from build123d import *

# Parameters (mm, degrees)
F0_R     = 18
F1_DEPTH = 10
F2_R     = 16
F3_DEPTH = 7
F4_R     = 4
F5_DEPTH = 25
F6_R     = 2


with BuildPart() as f1:
    # F0 (on Top) → F1 (new body)
    with BuildSketch(Plane.XY):
        Circle(F0_R)
    extrude(amount=F1_DEPTH)

    # F2 (on face) → F3 (cut)
    with BuildSketch(Plane.XY.offset(10)):
        Circle(F2_R)
    extrude(amount=-F3_DEPTH, mode=Mode.SUBTRACT)

    # F4 (on face) → F5 (cut)
    with BuildSketch(Plane(origin=(0, 0, 0), x_dir=(1, 0, 0), z_dir=(0, 0, -1))):
        Circle(F4_R)
    extrude(amount=-F5_DEPTH, mode=Mode.SUBTRACT)

    # F6
    f6_edges = [f1.edges().sort_by_distance(p)[0] for p in [
        (-18, 0, 0),
    ]]
    fillet(f6_edges, radius=F6_R)


solid = f1.part
Work out the finished part from the listing and answer in its coordinate system (mm). A direction names the side the tool comes from. Coordinates: 2 decimals unless noted, no trailing zeros. Write each loop counter-clockwise with the first axis right and the second up, starting at its lowest first coordinate (ties: lowest second). Pieces come first, ordered by that corner, then holes. Notation, with made-up numbers: M 34.5,58 L 62.5,58 A13 cw 62.5,63 Z; hole C 4.5,42.25 d9. An arc over 180 degrees is marked long. Write item = value, one per line.
1. Flat-ended cylindrical pins translate along their axes: pin 1 (3 mm diameter, centred on x = 6, z = 3, fed in from +Y); pin 2 (3 mm diameter, centred on x = 2.5, z = 4.5, fed in from +Y); pin 3 (4 mm diameter, centred on y = 7.5, z = 1.5, fed in from +X); pin 4 (5 mm diameter, centred on x = 0, y = 0, fed in from -Z). Find the tip coordinate at first contact, or state that the pin passes through.
Solution:
pin_1 = 17.43
pin_2 = 17.97
pin_3 = 17.12
pin_4 = through
2. The part is cut by section D-D (z = 1). Determine the outline of the cut face in (x, y).
Solution:
outline = C 0,0 d35.46; hole C 0,0 d8
3. The part is cut by section A-A (x = 0). Determine the outline of the cut face in (y, z).
Solution:
outline = M -18,2 A2 ccw -16,0 L -4,0 L -4,3 L -16,3 L -16,10 L -18,10 Z; M 4,0 L 16,0 A2 ccw 18,2 L 18,10 L 16,10 L 16,3 L 4,3 Z
4. For faces 1 (the face through (3, -3, 3)), 2 (the face through (-12, -11, 10)), determine the directions among +Z, -Z, +X, -X, +Y, -Y from which every point of the face is accessible in a straight line to the end or side of a thin tool.
Solution:
face_1 = +Z
face_2 = +Z, +X, -X, +Y, -Y
5. Determine the mould class of faces 3 (the face through (3, -3, 0)), 4 (the face through (-2.343, 17.847, 5.944)), 5 (the face through (-0.867, 3.905, 1.479)), 6 (the face through (-3.47, -15.62, 6.55)) for opening direction Y: released by +Y, released by -Y, zero draft, split by the parting line, or undercut.
Solution:
face_3 = zero draft
face_4 = split by the parting line
face_5 = undercut
face_6 = undercut
6. The part is cut by section C-C (z = 7.5). Determine the outline of the cut face in (x, y).
Solution:
outline = C 0,0 d36; hole C 0,0 d32
7. Straight lines are drawn through the part: line 1 (X direction, y = -6, z = 6.75); line 2 (Y direction, x = 0, z = 8); line 3 (Z direction, x = 10, y = 12). For each, find the intervals that lie inside material, in ascending order. Write a range as from..to.
Solution:
line_1 = -16.97..-14.83, 14.83..16.97
line_2 = -18..-16, 16..18
line_3 = 0..3
